Could you check a few things on this model? Use its own coordinates, in mm. Face numbers are marked on the shaded views. A direction names the side the tool comes from. Give positions to 0.01 mm unless a question says otherwise; leave off trailing zeros. Order: outer loops, then holes, each group sorted by start corner. A loop starts at its lowest first (then second) coordinate and runs counter-clockwise, first axis right, second up.
(1) Imagine slicing it at C-C, the plane y = -3.8. Write out the boundary of the cut face in (x, z).
(2) Imagine slicing it at A-A, the plane z = -10.5. Write out the boundary of the cut face in (x, y), then the cut area to 3 significant figures.
(3) Imagine slicing it at D-D, the plane z = -3.75. Write out the boundary of the cut face in (x, y), then the cut area to 3 significant figures.
(4) If I drill on probe 1 along X at (y, z) = (-2.05, -13); probe 2 along Y at (x, z) = (3, -14.5); probe 3 along X at (y, z) = (-4.3, -5.5), over which ranges is the centre line in solid material (lowest first)?
(5) On a 3-axis mill with a long thin cutter (end or side, diameter ignored), from which of +Z, -Z, +X, -X, +Y, -Y can I reach the whole of each face in a straight line? I mean the marked faces 1, 2, 3 and 4. Say none if no direction works.
(6) Will these pins go through, and if not, where does the flat tip stop? pin 1 (3 mm diameter, centred on x = -14, z = -3, fed in from +Y); pin 2 (6 mm diameter, centred on x = 1.5, z = -13, fed in from -Y); pin 3 (1.2 mm diameter, centred on x = 1, y = -4.5, fed in from -Z); pin 4 (5 mm diameter, centred on x = -13.5, z = -13, fed in from +Y).
(7) Imagine slicing it at B-B, the plane x = 3.5. Write out the boundary of the cut face in (y, z).
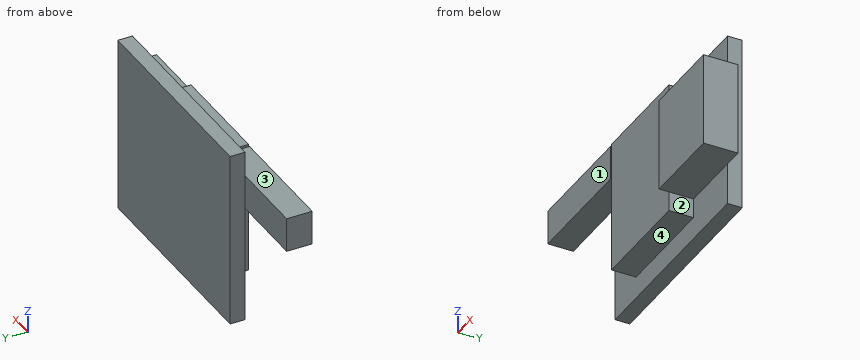
Autodesk Inventor part; units mm, degrees
ref_plane "РабПлоскость1" through (-8.75, -1.3, -1.3) normal (0, -1, 0) x (1, 0, 0)
ref_plane "YZ Plane" through (0, 0, 0) normal (1, 0, 0) x (0, 1, 0)
ref_plane "XZ Plane" through (0, 0, 0) normal (0, 1, 0) x (-1, 0, 0)
ref_plane "РабПлоскость1" through (-8.75, -1.3, -1.3) normal (0, -1, 0) x (1, 0, 0)
sketch "Эскиз1" plane through (-8.75, -1.3, -1.3) normal (0, -1, 0) x (1, 0, 0)
  line L0 (21.5, -15.4) -> (0, -15.4)
  line L1 (0, -15.4) -> (0, 2.6)
  line L2 (0, 2.6) -> (21.5, 2.6)
  line L3 (21.5, 2.6) -> (21.5, -15.4)
  point P0 (8.75, 1.3)
  point P1 (0, 2.6)
  dimension "d0" = 21.5
  dimension "d1" = 18
extrude "Выдавливание1" add sketch "Эскиз1" along normal blind 1.5
sketch "Эскиз2" plane through (-8.75, -2.8, -1.3) normal (0, -1, 0) x (1, 0, 0)
  line L0 (21.5, -15.4) -> (21.5, 2.6)
  line L1 (23.5, -1.65) -> (15, -1.65)
  line L2 (15, -1.65) -> (15, -11.15)
  line L3 (15, -11.15) -> (23.5, -11.15)
  line L4 (23.5, -11.15) -> (23.5, -1.65)
  point P0 (8.75, 1.3)
  point P1 (15, -6.4)
  point P2 (21.5, -6.4)
  dimension "d17" = 8.5
  dimension "d18" = 9.5
  dimension "d19" = 6.5
extrude "Выдавливание2" add sketch "Эскиз2" along normal blind 3.5
ref_plane "РабПлоскость2" through (-8.75, -1.3, -7.7) normal (0, 0, 1) x (1, 0, 0)
sketch "Эскиз4" plane through (-8.75, -2.8, -1.3) normal (0, -1, 0) x (1, 0, 0)
  line L0 (15, 0.35) -> (4, 0.35)
  line L1 (4, 0.35) -> (4, -13.15)
  line L2 (4, -13.15) -> (15, -13.15)
  line L3 (15, -13.15) -> (15, 0.35)
  line L4 (0, 2.6) -> (0, -15.4)
  point P0 (8.75, 1.3)
  point P1 (15, -6.4)
  point P2 (0, -6.4)
  dimension "d20" = 11
  dimension "d21" = 13.5
  dimension "d22" = 15
extrude "Выдавливание4" add sketch "Эскиз4" along normal blind 2.5
sketch "Эскиз5" plane through (-8.75, -2.8, -1.3) normal (0, -1, 0) x (1, 0, 0)
  line L0 (-1, -3.4) -> (4, -3.4)
  line L1 (4, -3.4) -> (4, 0.1)
  line L2 (4, 0.1) -> (-1, 0.1)
  line L3 (-1, 0.1) -> (-1, -3.4)
  line L4 (21.5, 2.6) -> (0, 2.6)
  line L5 (4, 0.35) -> (4, -13.15)
  point P0 (8.75, 1.3)
  point P1 (4, -1.65)
  point P2 (4, -6.4)
  dimension "d25" = 5
  dimension "d26" = 3.5
  dimension "d27" = 6
extrude "Выдавливание5" add sketch "Эскиз5" along normal blind 2.6
sketch "Эскиз6" plane through (-9.75, -2.8, -4.7) normal (-1, 0, 0) x (0, 0, 1)
  circle A0 centre (1.75, -1.3) radius 1
  line L0 (3.5, -2.6) -> (0, -2.6)
  line L1 (3.5, 0) -> (3.5, -2.6)
  line L2 (3.5, 0) -> (0, 0)
  line L3 (0, 0) -> (0, -2.6)
  point P0 (4.7, 2.8)
  point P1 (1.75, -2.6)
  point P2 (3.5, -1.3)
  dimension "d30" = 2
extrude "Выдавливание6" add sketch "Эскиз6" along normal blind 7 contours A0 | L0 L3 L2 L1
properties part number "ЛЦМК0000002.00.00.00.00.03"
Answer block:
1. outline: (-16.75, -4.7) - (-4.75, -4.7) - (-4.75, -14.45) - (6.25, -14.45) - (6.25, -12.45) - (14.75, -12.45) - (14.75, -2.95) - (6.25, -2.95) - (6.25, -0.95) - (-4.75, -0.95) - (-4.75, -1.2) - (-16.75, -1.2) - close
2. outline: (-8.75, -2.8) - (-4.75, -2.8) - (-4.75, -5.3) - (6.25, -5.3) - (6.25, -6.3) - (14.75, -6.3) - (14.75, -2.8) - (12.75, -2.8) - (12.75, -1.3) - (-8.75, -1.3) - close
2. area: 89.5 mm2
3. outline: (-16.75, -5.4) - (-4.75, -5.4) - (-4.75, -5.3) - (6.25, -5.3) - (6.25, -6.3) - (14.75, -6.3) - (14.75, -2.8) - (12.75, -2.8) - (12.75, -1.3) - (-8.75, -1.3) - (-8.75, -2.8) - (-16.75, -2.8) - close
3. area: 121 mm2
4. probe 1: x = -8.75 to 12.75
4. probe 2: y = -2.8 to -1.3
4. probe 3: x = -4.75 to 14.75
5. face 1: +Z, -Z, -X, -Y
5. face 2: -Z, +X, -Y
5. face 3: +Z, -X, -Y
5. face 4: -Z, +X, -X, -Y
6. pin 1: stops at y = -2.8
6. pin 2: stops at y = -5.3
6. pin 3: stops at z = -14.45
6. pin 4: passes through
7. outline: (-5.3, -14.45) - (-2.8, -14.45) - (-2.8, -16.7) - (-1.3, -16.7) - (-1.3, 1.3) - (-2.8, 1.3) - (-2.8, -0.95) - (-5.3, -0.95) - close
